Here's how the part is built. I have some questions about the finished solid (model axes, mm). Face numbers are marked on the shaded views. A direction names the side the tool comes from. Give positions to 0.01 mm unless a question says otherwise; leave off trailing zeros. Write each loop counter-clockwise with the first axis right and the second up, starting at its lowest first coordinate (ties: lowest second). Pieces come first, ordered by that corner, then holes. Notation, with made-up numbers: (-34.5, 11) - (-25.5, 11) arc R28 ccw to (-25.5, 39) - close; hole circle Ø5 at (48.5, 73.25). An arc over 180 degrees is marked (long way). Write each question's results on one line, items separated by ' | '. Start each with the question number.
Item 1: Suppose I cut it at B-B on x = -6.75. List the corners of the cut face in (y, z) for me.
Item 2: Which directions (+Z, -Z, +X, -X, +Y, -Y) give clear straight access to the entire face, cutting with the end or side of a thin tool? Please do the marked faces 4, 5, 6 and 7.
Item 3: Will these pins go through, and if not, where does the flat tip stop? P1, Ø3, axis at x = 3, y = 3, coming from the -Z side; P2, Ø0.8, axis at y = 3, z = 0.5, coming from the +X side; P3, Ø2, axis at x = 7.5, y = 0.5, coming from the +Z side.
Item 4: Suppose I cut it at D-D on y = 1.4. List the corners of the cut face in (x, z) for me, then the cut area to 3 significant figures.
Item 5: Suppose I cut it at A-A on y = 3.15. List the corners of the cut face in (x, z) for me, then the cut area to 3 significant figures.
Item 6: We'd pull the mould along Z, two halves only. Please class the marked faces 1, 2 and 3: +Z half, -Z half, draft (parallel to the pull), parting line (faces both ways), or undercut.
Item 7: Suppose I cut it at C-C on z = -4. List the corners of the cut face in (x, y) for me.
Item 8: Please list where these lines run through material, in increasing order: line 1 along X through (y, z) = (3.45, -0.75); line 2 along Y through (x, z) = (-2.25, 1.25); line 3 along Z through (x, y) = (5.75, 3.3).
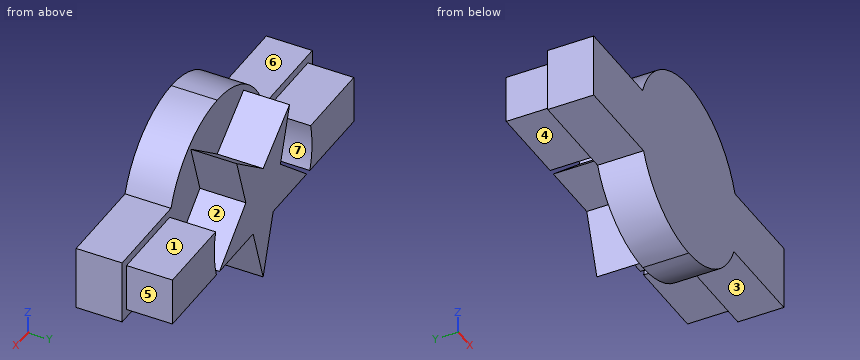
```python
from build123d import *

# Parameters (mm, degrees)
BOSS_EXTRUDE1_DEPTH   = 5
BOSS_EXTRUDE1_2_DEPTH = 5
BOSS_EXTRUDE2_DEPTH   = 2.5


with BuildPart() as part:
    # Sketch3 → Boss-Extrude1 (new body)
    with BuildSketch(Plane(origin=(0, 0, 0), x_dir=(1, 0, 0), z_dir=(0, 1, 0))):
        Polygon((1.026915579, 1.452751925), (0, 4.69), (0, -1.780366005), (2.703467563, -3.832409573), (1.768831042, -0.886061948), (4.459328632, 1.452751925), align=None)
    extrude(amount=BOSS_EXTRUDE1_DEPTH)



with BuildPart() as body_2:
    # Sketch3 → Boss-Extrude1 2 (new body)
    with BuildSketch(Plane(origin=(0, 0, 0), x_dir=(1, 0, 0), z_dir=(0, 1, 0))):
        with BuildLine():
            Line((9.280338467, 1.452751925), (4.784298469, 1.452751925))
            ThreePointArc((4.784298469, 1.452751925), (4.997850706, 0.146588935), (4.861220275, -1.16984505))
            Line((4.861220275, -1.16984505), (9.280338467, -1.16984505))
            Line((9.280338467, -1.16984505), (9.280338467, 1.452751925))
        make_face()
    extrude(amount=BOSS_EXTRUDE1_2_DEPTH)


with BuildPart() as part_1:
    add(part.part)

    add(body_2.part)  # Boss-Extrude2 merges body 2
    # Sketch3_3 → Boss-Extrude2 (add)
    with BuildSketch(Plane(origin=(0, 0, 0), x_dir=(1, 0, 0), z_dir=(0, 1, 0))):
        with BuildLine():
            ThreePointArc((4.784298469, 1.452751925), (4.709427631, 1.679670023), (4.623800938, 1.902751925))
            ThreePointArc((4.623800938, 1.902751925), (2.782646256, 4.154140081), (0, 5))
            Line((0, 5), (0, 4.69))
            Line((0, 4.69), (1.026915579, 1.452751925))
            Line((1.026915579, 1.452751925), (4.459328632, 1.452751925))
            Line((4.459328632, 1.452751925), (1.768831042, -0.886061948))
            Line((1.768831042, -0.886061948), (2.703467563, -3.832409573))
            Line((2.703467563, -3.832409573), (0, -1.780366005))
            Line((0, -1.780366005), (0, -5))
            ThreePointArc((0, -5), (2.906955, -4.068121511), (4.730338467, -1.61984505))
            ThreePointArc((4.730338467, -1.61984505), (4.801054548, -1.396379328), (4.861220275, -1.16984505))
            ThreePointArc((4.861220275, -1.16984505), (4.997850706, 0.146588935), (4.784298469, 1.452751925))
        make_face()
        with BuildLine():
            Line((9.730338467, -1.61984505), (9.730338467, 1.902751925))
            Line((9.730338467, 1.902751925), (4.623800938, 1.902751925))
            ThreePointArc((4.623800938, 1.902751925), (4.709427631, 1.679670023), (4.784298469, 1.452751925))
            Line((4.784298469, 1.452751925), (9.280338467, 1.452751925))
            Line((9.280338467, 1.452751925), (9.280338467, -1.16984505))
            Line((9.280338467, -1.16984505), (4.861220275, -1.16984505))
            ThreePointArc((4.861220275, -1.16984505), (4.801054548, -1.396379328), (4.730338467, -1.61984505))
            Line((4.730338467, -1.61984505), (9.730338467, -1.61984505))
        make_face()
    extrude(amount=BOSS_EXTRUDE2_DEPTH)

    # Mirror1: part across plane


with BuildPart() as part_2:
    add(part_1.part)
    add(part_1.part.mirror(Plane(origin=(0, 0, 0), x_dir=(0, 0, 1), z_dir=(1, 0, 0))))


solid = part_2.part
```
Checked values:
1) outline: (0, -1.9) - (2.5, -1.9) - (2.5, -1.45) - (5, -1.45) - (5, 1.17) - (2.5, 1.17) - (2.5, 1.62) - (0, 1.62) - close
2) face 4: -Z, -X, +Y | face 5: +Z, -Z, +X, +Y | face 6: +Z, -X, +Y, -Y | face 7: +Y
3) P1: stops at z = -4.74 | P2: stops at x = 9.28 | P3: stops at z = 1.62
4) outline: (-9.73, -1.9) - (-4.62, -1.9) arc R5 ccw to (4.62, -1.9) - (9.73, -1.9) - (9.73, 1.62) - (4.73, 1.62) arc R5 ccw to (-4.73, 1.62) - (-9.73, 1.62) - close | area: 113 mm^2
5) outline: (-9.28, -1.45) - (-4.78, -1.45) arc R5 cw to (-4.86, 1.17) - (-9.28, 1.17) - close; (-4.46, -1.45) - (-1.03, -1.45) - (0, -4.69) - (1.03, -1.45) - (4.46, -1.45) - (1.77, 0.89) - (2.7, 3.83) - (0, 1.78) - (-2.7, 3.83) - (-1.77, 0.89) - close; (4.78, -1.45) - (9.28, -1.45) - (9.28, 1.17) - (4.86, 1.17) arc R5 cw to start | area: 48.3 mm^2
6) face 1: +Z half | face 2: undercut | face 3: -Z half
7) outline: (-3, 0) - (3, 0) - (3, 2.5) - (0.22, 2.5) - (0.22, 5) - (-0.22, 5) - (-0.22, 2.5) - (-3, 2.5) - close
8) line 1: x = -9.28 to -4.94, -3.65 to 3.65, 4.94 to 9.28 | line 2: y = 0 to 2.5 | line 3: z = -1.45 to 1.17
